Read the model definition and answer for the solid it produces. Units are mm, in the model's axes. A direction names the side the tool comes from. Coordinates: 2 decimals unless noted, no trailing zeros. Write each loop counter-clockwise with the first axis right and the second up, starting at its lowest first coordinate (ties: lowest second). Pieces come first, ordered by that corner, then holes. Notation, with made-up numbers: (4.5, 82) - (18.5, 82) arc R9 ccw to (18.5, 91) - close; hole circle Ø8 at (-16, -36.5). An arc over 180 degrees is marked (long way). Return JSON: item names as keys, results as strings.
```python
from build123d import *

# Parameters (mm, degrees)
SKETCH1_R           = 30
BOSS_EXTRUDE1_DEPTH = 2
SKETCH2_R           = 24.5
BOSS_EXTRUDE2_DEPTH = 6
SKETCH3_R           = 30
BOSS_EXTRUDE3_DEPTH = 2
SKETCH4_R           = 11
SKETCH4_R_2         = 2.25
CUT_EXTRUDE1_DEPTH  = 2
SKETCH5_R           = 2.25
CUT_EXTRUDE2_DEPTH  = 27
SKETCH6_R           = 1.75
CUT_EXTRUDE3_DEPTH  = 27
SKETCH7_R           = 11
CUT_EXTRUDE4_DEPTH  = 2


with BuildPart() as part:
    # Sketch1 → Boss-Extrude1 (new body)
    with BuildSketch(Plane(origin=(0, 0, 0), x_dir=(1, 0, 0), z_dir=(0, 1, 0))):
        Circle(SKETCH1_R)
    extrude(amount=BOSS_EXTRUDE1_DEPTH)

    # Sketch2 → Boss-Extrude2 (add)
    with BuildSketch(Plane(origin=(0, 2, 0), x_dir=(1, 0, 0), z_dir=(0, 1, 0))):
        Circle(SKETCH2_R)
    extrude(amount=BOSS_EXTRUDE2_DEPTH)

    # Sketch3 → Boss-Extrude3 (add)
    with BuildSketch(Plane(origin=(0, 8, 0), x_dir=(1, 0, 0), z_dir=(0, 1, 0))):
        Circle(SKETCH3_R)
    extrude(amount=BOSS_EXTRUDE3_DEPTH)

    # Sketch4 → Cut-Extrude1 (cut)
    with BuildSketch(Plane(origin=(0, 10, 0), x_dir=(1, 0, 0), z_dir=(0, 1, 0))):
        Circle(SKETCH4_R)
        Circle(SKETCH4_R_2, mode=Mode.SUBTRACT)
    extrude(amount=-CUT_EXTRUDE1_DEPTH, mode=Mode.SUBTRACT)

    # Sketch5 → Cut-Extrude2 (cut)
    with BuildSketch(Plane(origin=(0, 10, 0), x_dir=(1, 0, 0), z_dir=(0, 1, 0))):
        Circle(SKETCH5_R)
    extrude(amount=-CUT_EXTRUDE2_DEPTH, mode=Mode.SUBTRACT)

    # Sketch6 → Cut-Extrude3 (cut)
    with BuildSketch(Plane(origin=(0, 8, 0), x_dir=(1, 0, 0), z_dir=(0, 1, 0))):
        with Locations((0, 7)):
            Circle(SKETCH6_R)
        with Locations((7, 0)):
            Circle(SKETCH6_R)
        with Locations((0, -7)):
            Circle(SKETCH6_R)
        with Locations((-7, 0)):
            Circle(SKETCH6_R)
    extrude(amount=-CUT_EXTRUDE3_DEPTH, mode=Mode.SUBTRACT)

    # Sketch7 → Cut-Extrude4 (cut)
    with BuildSketch(Plane.XZ):
        Circle(SKETCH7_R)
    extrude(amount=-CUT_EXTRUDE4_DEPTH, mode=Mode.SUBTRACT)


solid = part.part
```
(1) Flat-ended cylindrical pins translate along their axes: P1, Ø4.5, axis at x = 0, z = -7, coming from the -Y side; P2, Ø4, axis at x = 0, z = 7, coming from the +Y side; P3, Ø6, axis at x = -14.5, y = 6, coming from the +Z side. Find the tip coordinate at first contact, or state that the pin passes through.
Answer:
{"P1": "y = 2", "P2": "y = 8", "P3": "z = 27.38"}
(2) A cutting plane is placed at A-A (z = 0). State how many separate pieces and enclosed holes the cut face has, and give its area (3 significant figures).
Answer:
{"separate pieces": "4", "enclosed holes": "0", "area": "377 mm²"}
(3) Which of the six approach directions +Z, -Z, +X, -X, +Y, -Y give full straight-line access (tool end or side, diameter ignored) to faces 4 (the face through (-2.38, 0.99, -10.74)), 5 (the face through (13, 0, 0)), 6 (the face through (-2.38, 9.01, 10.74)), 7 (the face through (-25, 2, 0)), 8 (the face through (-0.38, 5.04, -5.29))?
Answer:
{"face 4": "-Y", "face 5": "+Z, -Z, +X, -X, -Y", "face 6": "+Y", "face 7": "none", "face 8": "+Y, -Y"}
(4) A cutting plane is placed at C-C (x = -7). Determine the outline of the cut face in (y, z), and give its area (3 significant figures).
Answer:
{"outline": "(0, -29.17) - (2, -29.17) - (2, -23.48) - (8, -23.48) - (8, -29.17) - (10, -29.17) - (10, -8.49) - (8, -8.49) - (8, -1.75) - (2, -1.75) - (2, -8.49) - (0, -8.49) - close; (0, 8.49) - (2, 8.49) - (2, 1.75) - (8, 1.75) - (8, 8.49) - (10, 8.49) - (10, 29.17) - (8, 29.17) - (8, 23.48) - (2, 23.48) - (2, 29.17) - (0, 29.17) - close", "area": "426 mm²"}
(5) Straight lines are drawn through the part: line 1 (X direction, y = 4.6, z = 0); line 2 (Y direction, x = -22, z = 11); line 3 (Z direction, x = 0, y = 9.15). For each, find the intervals that lie inside material, in ascending order. Write a range as from..to.
Answer:
{"line 1": "-24.5..-8.75, -5.25..-2.25, 2.25..5.25, 8.75..24.5", "line 2": "0..2, 8..10", "line 3": "-30..-11, 11..30"}
(6) A cutting plane is placed at D-D (y = 3.25). Determine the outline of the cut face in (x, z).
Answer:
{"outline": "circle Ø49 at (0, 0); hole circle Ø3.5 at (-7, 0); hole circle Ø4.5 at (0, 0); hole circle Ø3.5 at (0, -7); hole circle Ø3.5 at (0, 7); hole circle Ø3.5 at (7, 0)"}
(7) Determine the mould class of faces 1 (the face through (-0.29, 5.04, -2.23)), 2 (the face through (-25, 8, 0)), 3 (the face through (-29.97, 8.99, -1.32)) for opening direction X: +X half, -X half, draft (parallel to the pull), parting line (faces both ways), or undercut.
Answer:
{"face 1": "undercut", "face 2": "draft", "face 3": "parting line"}
